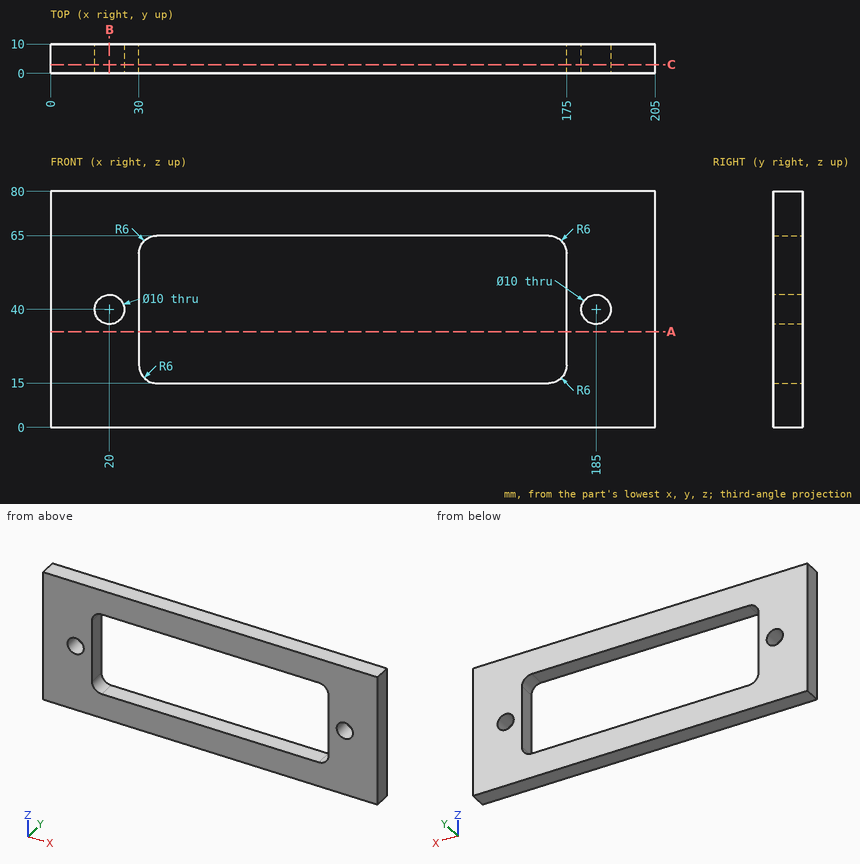
For this review, use the dimensioned drawing (mm, ordinates from the lowest corner) and the shaded views. Give positions to 0.01 mm unless a question says otherwise; leave off trailing zeros. Loops run counter-clockwise (first coordinate to the right, second up) from the corner with the lowest first, then second, coordinate; pieces in that order, holes last.
Item 1: Take a section at A-A, the plane z = 32.5. State the section outline as (x, y) points.
Item 2: Take a section at C-C, the plane y = 3. State the section outline as (x, z) points.
Item 3: For line 1 along Z through (x, y) = (89, 4.25); line 2 along Z through (x, y) = (20, 5.5); line 3 along X through (y, z) = (6.5, 29), list the stretches that pass through material, from the lowest coordinate up.
Item 4: Insertion check: pin 1 (9 mm diameter, centred on x = 185, z = 40, fed in from -Y). The pin has a flat end and moves straight along its axis. Give the tip position at first contact, or say it passes through.
Item 5: Take a section at B-B, the plane x = 20. State the section outline as (y, z) points, and give its area (3 significant figures).
Calculated:
1. outline: (0, 0) - (30, 0) - (30, 10) - (0, 10) - close; (175, 0) - (205, 0) - (205, 10) - (175, 10) - close
2. outline: (0, 0) - (205, 0) - (205, 80) - (0, 80) - close; hole circle Ø10 at (20, 40); hole (30, 21) arc R6 ccw to (36, 15) - (169, 15) arc R6 ccw to (175, 21) - (175, 59) arc R6 ccw to (169, 65) - (36, 65) arc R6 ccw to (30, 59) - close; hole circle Ø10 at (185, 40)
3. line 1: z = 0 to 15, 65 to 80
3. line 2: z = 0 to 35, 45 to 80
3. line 3: x = 0 to 30, 175 to 205
4. pin 1: passes through
5. outline: (0, 0) - (10, 0) - (10, 35) - (0, 35) - close; (0, 45) - (10, 45) - (10, 80) - (0, 80) - close
5. area: 700 mm2
